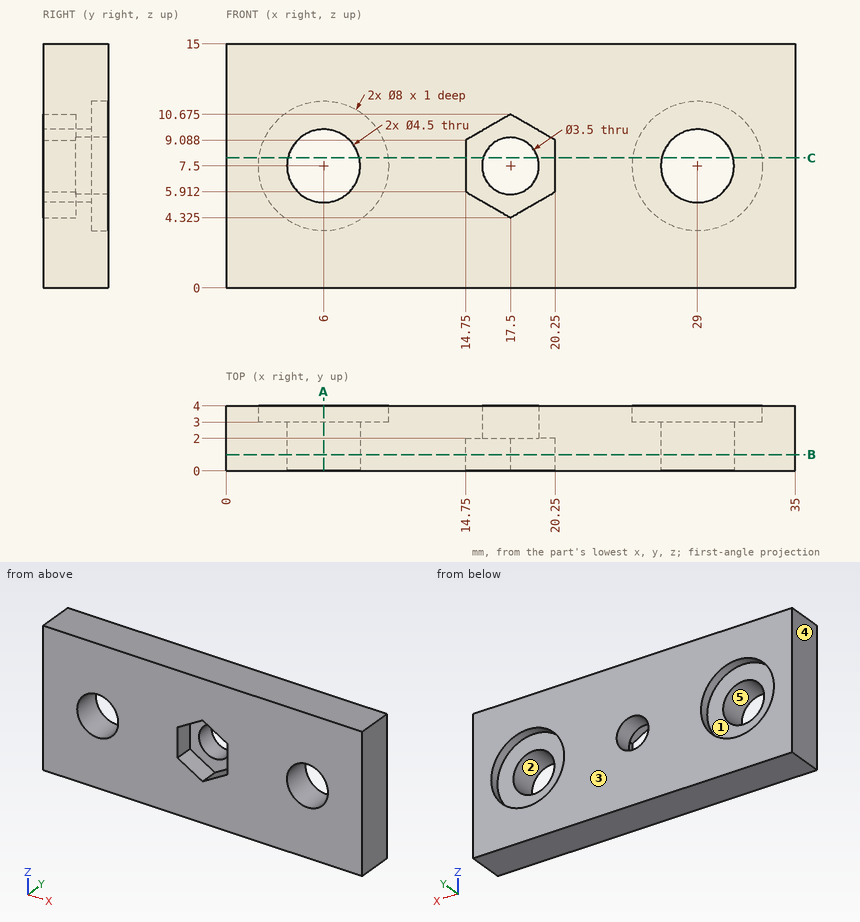
Drawing for the job (mm, zero at the part's lowest x, y, z). A direction names the side the tool comes from. Coordinates: 2 decimals unless noted, no trailing zeros. Write each loop counter-clockwise with the first axis right and the second up, starting at its lowest first coordinate (ties: lowest second). Pieces come first, ordered by that corner, then holes. Notation, with made-up numbers: (35, 25.25) - (84, 25.25) arc R25 cw to (84, 49.25) - close; hole circle Ø6 at (-37.5, 78). An arc over 180 degrees is marked (long way). Write each question's results on one line, items separated by ' | '. Start each with the question number.
1) Mould opens along X. For the marked faces 3, 4 and 5 say: pulls with the +X half, pulls with the -X half, needs draft (parallel to the pull), parting line crosses it, or undercut.
2) Cut at A-A (x = 6). Write the cut outline in (y, z), then the cut area to 3 significant figures.
3) Flat gauge pins, fed straight in: P1, Ø4, axis at x = 6, z = 7.5, coming from the -Y side; P2, Ø7, axis at x = 6, z = 7.5, coming from the +Y side; P3, Ø4, axis at x = 17.5, z = 7.5, coming from the -Y side. Where does each tip first touch, or does it go through?
4) Cut at B-B (y = 1). Count the separate pieces of the cut face and the enclosed holes in it, then the cut area to 3 significant figures.
5) 3-axis set-ups, long thin cutter, end or side, ignore diameter. For the marked faces 1 and 2: which of +Z, -Z, +X, -X, +Y, -Y reach the whole face in a straight line?
6) Probe line 1 along Z through (x, y) = (6, 0.9); line 2 along Z through (x, y) = (17.5, 3.55); line 3 along X through (y, z) = (3.3, 9.5) (1 decimal). List the from-to ranges inside material, lowest first. Write a range as from..to.
7) Cut at C-C (z = 8). Write the cut outline in (x, y).
Returned:
1) face 3: needs draft | face 4: pulls with the -X half | face 5: undercut
2) outline: (0, 0) - (4, 0) - (4, 3.5) - (3, 3.5) - (3, 5.25) - (0, 5.25) - close; (0, 9.75) - (3, 9.75) - (3, 11.5) - (4, 11.5) - (4, 15) - (0, 15) - close | area: 38.5 mm^2
3) P1: through | P2: y = 3 | P3: y = 2
4) separate pieces: 1 | enclosed holes: 3 | area: 467 mm^2
5) face 1: +Y | face 2: +Y, -Y
6) line 1: 0..5.25, 9.75..15 | line 2: 0..5.75, 9.25..15 | line 3: 0..2.5, 9.5..25.5, 32.5..35
7) outline: (0, 0) - (3.81, 0) - (3.81, 3) - (2.03, 3) - (2.03, 4) - (0, 4) - close; (8.19, 0) - (14.75, 0) - (14.75, 2) - (15.82, 2) - (15.82, 4) - (9.97, 4) - (9.97, 3) - (8.19, 3) - close; (19.18, 2) - (20.25, 2) - (20.25, 0) - (26.81, 0) - (26.81, 3) - (25.03, 3) - (25.03, 4) - (19.18, 4) - close; (31.19, 0) - (35, 0) - (35, 4) - (32.97, 4) - (32.97, 3) - (31.19, 3) - close
